The listing builds one solid part. Answer for the finished solid, in the listing's coordinates (mm). A direction names the side the tool comes from. Round coordinates to 2 decimals unless told otherwise and drop trailing zeros. Write each loop counter-clockwise with the first axis right and the second up, starting at its lowest first coordinate (ties: lowest second). Pieces come first, ordered by that corner, then holes. Notation, with made-up numbers: (75.5, 63.5) - (95.5, 63.5) arc R6 cw to (95.5, 68.5) - close; hole circle Ø10 at (30.25, 63.25). An arc over 180 degrees is marked (long way). Answer as CSV lines item,"result". Start each with the question number.
Item 1: A cutting plane is placed at A-A on y = 22.5. Determine the outline of the cut face in (x, z) (3 decimals), and give its area (4 significant figures).
Item 2: Flat-ended cylindrical pins translate along their axes: pin 1 (1.5 mm diameter, centred on x = 92, z = 2.5, fed in from -Y); pin 2 (2 mm diameter, centred on x = 63.875, y = 42.125, fed in from +Z). Find the tip coordinate at first contact, or state that the pin passes through.
Item 3: A cutting plane is placed at B-B on x = 15. Determine the outline of the cut face in (y, z), and give its area (4 significant figures).
Item 4: A cutting plane is placed at C-C on x = 87.5. Determine the outline of the cut face in (y, z) (3 decimals).
Item 5: Straight lines are drawn through the part: line 1 along Y through (x, z) = (79.5, 2.25) (3 decimals); line 2 along Y through (x, z) = (15, 2.45); line 3 along Y through (x, z) = (104.5, 0.95). For each, find the intervals that lie inside material, in ascending order. Write a range as [from, to].
Item 6: For a pull along Y with two mould halves and no side action, classify faces 4 (the flat face through (90, 23, 5)), 5 (the flat face through (69, 4, 2)), 6 (the cylindrical face through (14.339, 27.023, 2.465)), 7 (the cylindrical face through (0.9, 44.14, 2.54)) as pulls with the +Y half, pulls with the -Y half, needs draft (parallel to the pull), parting line crosses it, or undercut.
Item 7: A cutting plane is placed at D-D on z = 2.05. State how many separate pieces and enclosed holes the cut face has, and give its area (3 significant figures).
Item 8: Which of the six approach directions +Z, -Z, +X, -X, +Y, -Y give full straight-line access (tool end or side, diameter ignored) to faces 1 (the flat face through (90, 23, 0)), 2 (the flat face through (83, 0, 2)), 3 (the flat face through (84, 6.575, 2))?
```python
from build123d import *

# Parameters (mm, degrees)
SKETCH1_R           = 3.05
SKETCH1_R_2         = 2.55
SKETCH1_R_3         = 1.3
SKETCH1_W           = 30
SKETCH1_H           = 5
BOSS_EXTRUDE1_DEPTH = 5
FILLET1_R           = 3


with BuildPart() as part:
    # Sketch1 → Boss-Extrude1 (new body)
    with BuildSketch(Plane.XY):
        Polygon((183, -12), (183, 45), (0, 45), (0, 0), (165.78, 0), (177.78, -12), align=None)
        with Locations((15, 30)):
            Circle(SKETCH1_R, mode=Mode.SUBTRACT)
        with Locations((168, 30)):
            Circle(SKETCH1_R, mode=Mode.SUBTRACT)
        with Locations((119.125, 29.5)):
            Circle(SKETCH1_R_2, mode=Mode.SUBTRACT)
        with Locations((119.125, 22.5)):
            Circle(SKETCH1_R_2, mode=Mode.SUBTRACT)
        with Locations((119.125, 15.5)):
            Circle(SKETCH1_R_2, mode=Mode.SUBTRACT)
        with Locations((63.875, 42.125)):
            Circle(SKETCH1_R_3, mode=Mode.SUBTRACT)
        with Locations((104.125, 42.125)):
            Circle(SKETCH1_R_3, mode=Mode.SUBTRACT)
        with Locations((104.125, 2.875)):
            Circle(SKETCH1_R_3, mode=Mode.SUBTRACT)
        with Locations((63.875, 2.875)):
            Circle(SKETCH1_R_3, mode=Mode.SUBTRACT)
        with Locations((84, 40.925)):
            Rectangle(SKETCH1_W, SKETCH1_H, mode=Mode.SUBTRACT)
        with Locations((84, 4.075)):
            Rectangle(SKETCH1_W, SKETCH1_H, mode=Mode.SUBTRACT)
    extrude(amount=BOSS_EXTRUDE1_DEPTH)

    # Fillet1
    fillet1_edges = [part.edges().sort_by_distance(p)[0] for p in [
        (0, 0, 2.5),
        (0, 45, 2.5),
        (183, 45, 2.5),
        (183, -12, 2.5),
        (177.78, -12, 2.5),
        (165.78, 0, 2.5),
    ]]
    fillet(fillet1_edges, radius=FILLET1_R)


solid = part.part
```
Geometry says:
1,outline,"(0, 0) - (116.575, 0) - (116.575, 5) - (0, 5) - close; (121.675, 0) - (183, 0) - (183, 5) - (121.675, 5) - close"
1,area,"889.5 mm^2"
2,pin 1,"stops at y = 0"
2,pin 2,"passes through"
3,outline,"(0, 0) - (26.95, 0) - (26.95, 5) - (0, 5) - close; (33.05, 0) - (45, 0) - (45, 5) - (33.05, 5) - close"
3,area,"194.5 mm^2"
4,outline,"(0, 0) - (1.575, 0) - (1.575, 5) - (0, 5) - close; (6.575, 0) - (38.425, 0) - (38.425, 5) - (6.575, 5) - close; (43.425, 0) - (45, 0) - (45, 5) - (43.425, 5) - close"
5,line 1,"y = [0, 1.575], [6.575, 38.425], [43.425, 45]"
5,line 2,"y = [0, 26.95], [33.05, 45]"
5,line 3,"y = [0, 1.63], [4.12, 40.88], [43.37, 45]"
6,face 4,"needs draft"
6,face 5,"undercut"
6,face 6,"undercut"
6,face 7,"pulls with the +Y half"
7,separate pieces,"1"
7,enclosed holes,"11"
7,area,"7,920 mm^2"
8,face 1,"-Z, +X, -X, +Y, -Y"
8,face 2,"+Z, -Z, -X, -Y"
8,face 3,"+Z, -Z"
